Design review of the part built by this model. Coordinates are the model's own, in mm. A direction names the side the tool comes from. Round coordinates to 2 decimals unless told otherwise and drop trailing zeros. Order: outer loops, then holes, each group sorted by start corner. A loop starts at its lowest first (then second) coordinate and runs counter-clockwise, first axis right, second up. Notation, with made-up numbers: M 70.5,79.5 L 117.5,79.5 A11 cw 117.5,96.5 Z; hole C 58.5,89.25 d10. An arc over 180 degrees is marked long. Write each question's results on one line, items separated by ' | '. Start each with the question number.
Item 1: Machinability: for faces 4 (the cylindrical face through (0.26, 3.21, 0.3)), 5 (the flat face through (0, 0, 17)), 6 (the cylindrical face through (0.26, 3.21, 16.7)), which of the approach directions +Z, -Z, +X, -X, +Y, -Y give a long, thin tool a straight path to every point of the face, cutting with its end or side? Answer none if there is none.
Item 2: The part is to be moulded in two halves that separate along Z. For faces 1 (the cylindrical face through (-0.26, -3.21, 0.3)), 2 (the cylindrical face through (-0.26, -3.21, 16.7)), 3 (the cylindrical face through (-18.5, 0.2, 8.4)), say which applies: +Z half, -Z half, draft (parallel to the pull), parting line (faces both ways), or undercut.
Item 3: Clearance check with flat-ended pins moving along their axes: pin 1 (1 mm diameter, centred on x = 0.5, z = 8.5, fed in from +Y); pin 2 (2 mm diameter, centred on y = 1.5, z = 4, fed in from +X); pin 3 (3 mm diameter, centred on x = -10, z = 15, fed in from +Y). State where each tip first meets the part, or that it passes through.
Item 4: Wall thickness on line 1 (Y direction, x = -14.5, z = 5); line 2 (X direction, y = 1, z = 13); line 3 (Y direction, x = -5.5, z = 1.25): over which ranges is each line inside the solid? List them lowest first. Write a range as [from, to].
Item 5: Take a section at A-A, the plane z = 13.5. Write out the cut boundary in (x, y), plus the area to 3 significant figures.
```python
from build123d import *

# Parameters (mm, degrees)
RESSALTO_EXTRUS_O1_DEPTH = 17
FILETE1_R                = 1


with BuildPart() as part:
    # Esboço1 → Ressalto-extrusão1 (new body)
    with BuildSketch(Plane.XY):
        with BuildLine():
            Line((-14.947871578, 3.723044087), (15.052128422, 3.276179478))
            ThreePointArc((15.052128422, 3.276179478), (18.499611782, -0.275560726), (14.947871578, -3.723044087))
            Line((14.947871578, -3.723044087), (-15.052128422, -3.276179478))
            ThreePointArc((-15.052128422, -3.276179478), (-18.499611782, 0.275560726), (-14.947871578, 3.723044087))
        make_face()
    extrude(amount=RESSALTO_EXTRUS_O1_DEPTH)

    # Filete1
    filete1_edges = [part.edges().sort_by_distance(p)[0] for p in [
        (18.499611782, -0.275560726, 17),
        (0.052128422, 3.499611782, 17),
        (-18.499611782, 0.275560726, 17),
        (0.052128422, 3.499611782, 0),
        (18.499611782, -0.275560726, 0),
        (-0.052128422, -3.499611782, 0),
        (-18.499611782, 0.275560726, 0),
        (-0.052128422, -3.499611782, 17),
    ]]
    fillet(filete1_edges, radius=FILETE1_R)


solid = part.part
```
Results list:
1) face 4: -Z, +X, +Y | face 5: +Z, +X, -X, +Y, -Y | face 6: +Z, +X, +Y
2) face 1: -Z half | face 2: +Z half | face 3: draft
3) pin 1: y = 3.5 | pin 2: x = 18.42 | pin 3: y = 3.67
4) line 1: [-3.28, 3.72] | line 2: [-18.41, 18.28] | line 3: [-3.42, 3.58]
5) outline: M -15.05,-3.28 L 14.95,-3.72 A3.5 ccw 15.05,3.28 L -14.95,3.72 A3.5 ccw Z | area: 249 mm²
